The figure shows three views and two pictorial views of one solid part (mm, origin at its lowest corner). Answer the questions. Coordinates: 2 decimals unless noted, no trailing zeros. Write each loop counter-clockwise with the first axis right and the second up, starting at its lowest first coordinate (ties: lowest second). Pieces come first, ordered by that corner, then holes.
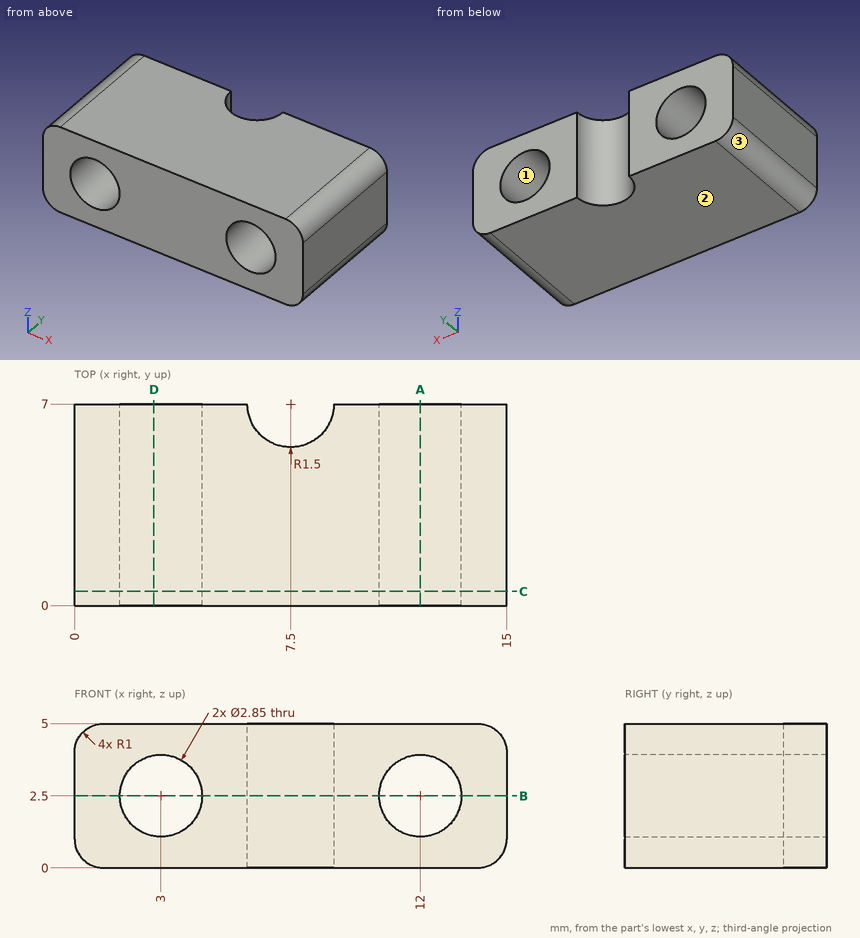
Q1. The part is cut by section D-D, the plane x = 2.75. Write down the section's boundary in (y, z).
Answers below:
outline: (0, 0) - (7, 0) - (7, 1.1) - (0, 1.1) - close; (0, 3.9) - (7, 3.9) - (7, 5) - (0, 5) - close
Q2. Find the intervals of material crossed by probe 1 along X at (y, z) = (2, 2.5) (3 decimals); probe 2 along X at (y, z) = (3, 1.25); probe 3 along Z at (x, y) = (11.75, 5.75), in increasing order.
Answers below:
probe 1: x = 0 to 1.575, 4.425 to 10.575, 13.425 to 15
probe 2: x = 0 to 2.32, 3.68 to 11.32, 12.68 to 15
probe 3: z = 0 to 1.1, 3.9 to 5
Q3. The part is cut by section A-A, the plane x = 12. Write down the section's boundary in (y, z) (3 decimals), then the cut area to 4 significant figures.
Answers below:
outline: (0, 0) - (7, 0) - (7, 1.075) - (0, 1.075) - close; (0, 3.925) - (7, 3.925) - (7, 5) - (0, 5) - close
area: 15.05 mm2
Q4. Determine the mould class of the marked faces 1, 2 and 3 for opening direction X: released by +X, released by -X, zero draft, split by the parting line, or undercut.
Answers below:
face 1: undercut
face 2: zero draft
face 3: released by -X
Q5. The part is cut by section C-C, the plane y = 0.5. Write down the section's boundary in (x, z) (3 decimals), then the cut area to 3 significant figures.
Answers below:
outline: (0, 1) arc R1 ccw to (1, 0) - (14, 0) arc R1 ccw to (15, 1) - (15, 4) arc R1 ccw to (14, 5) - (1, 5) arc R1 ccw to (0, 4) - close; hole circle Ø2.85 at (3, 2.5); hole circle Ø2.85 at (12, 2.5)
area: 61.4 mm2
Q6. The part is cut by section B-B, the plane z = 2.5. Write down the section's boundary in (x, y) (3 decimals).
Answers below:
outline: (0, 0) - (1.575, 0) - (1.575, 7) - (0, 7) - close; (4.425, 0) - (10.575, 0) - (10.575, 7) - (9, 7) arc R1.5 cw to (6, 7) - (4.425, 7) - close; (13.425, 0) - (15, 0) - (15, 7) - (13.425, 7) - close
Q7. Given pin 1 (1.5 mm diameter, centred on y = 6, z = 4, fed in from -X); pin 2 (1.7 mm diameter, centred on x = 12, z = 2.5, fed in from -Y) (3 decimals), each flat-ended and moving along its own axis, determine where each tip first touches the part or whether it passes through.
Answers below:
pin 1: stops at x = 0
pin 2: passes through
